```python
from build123d import *

# Parameters (mm, degrees)
SKETCH1_R           = 2.5
BOSS_EXTRUDE1_DEPTH = 15
CUT_EXTRUDE1_DEPTH  = 10


with BuildPart() as part:
    # Sketch1 → Boss-Extrude1 (new body, symmetric)
    with BuildSketch(Plane.XY):
        Circle(SKETCH1_R)
    extrude(amount=BOSS_EXTRUDE1_DEPTH, both=True)

    # Sketch2 → Cut-Extrude1 (cut)
    with BuildSketch(Plane(origin=(0, 0, -15), x_dir=(-1, 0, 0), z_dir=(0, 0, -1))):
        with BuildLine():
            Line((-0.5, -2.449489743), (-0.5, -1.949489743))
            Line((-0.5, -1.949489743), (0.5, -1.949489743))
            Line((0.5, -1.949489743), (0.5, -2.449489743))
            ThreePointArc((0.5, -2.449489743), (0, -2.5), (-0.5, -2.449489743))
        make_face()
    extrude(amount=-CUT_EXTRUDE1_DEPTH, mode=Mode.SUBTRACT)


solid = part.part
```
Input: part model. Units: mm. Frame: model coordinates. Coordinates: 2 decimals unless noted, no trailing zeros. Order: outer loops, then holes, each group sorted by start corner. A loop starts at its lowest first (then second) coordinate and runs counter-clockwise, first axis right, second up. Notation, with made-up numbers: (41.5, 12) - (84.5, 12) arc R27 ccw to (84.5, 32) - close; hole circle Ø4 at (79, 17.5). An arc over 180 degrees is marked (long way). Put each result on its own line as item: value.
1. Line query: line 1 along Z through (x, y) = (-0.2, -2.05); line 2 along X through (y, z) = (-2.1, -12); line 3 along Y through (x, z) = (0.1, 3). Output: solid intervals per line, ascending.
Report:
line 1: z = -5 to 15
line 2: x = -1.36 to -0.5, 0.5 to 1.36
line 3: y = -2.5 to 2.5
2. Contact query for flat-ended pins moving along their axis: pin 1 Ø0.6 at (x, y) = (0, -2.5) entering from -Z; pin 2 Ø0.8 at (x, z) = (0, -8) entering from -Y. Output: stop coordinate, or through.
Report:
pin 1: stops at z = -5
pin 2: stops at y = -1.95
3. Cut plane A-A on x = 0.2. Return the cut outline in (y, z), then the cut area to 3 significant figures.
Report:
outline: (-2.49, -5) - (-1.95, -5) - (-1.95, -15) - (2.49, -15) - (2.49, 15) - (-2.49, 15) - close
area: 144 mm2
4. Cut plane D-D on x = 1.4. Return the cut outline in (y, z).
Report:
outline: (-2.07, -15) - (2.07, -15) - (2.07, 15) - (-2.07, 15) - close
5. Draft query along X for faces 1 (the face through (-0.54, -2.44, 0.21)), 2 (the face through (0, -1.949, -10)), 3 (the face through (0, 0, -15)). Return one class per face: pulls with the +X half, pulls with the -X half, needs draft (parallel to the pull), parting line crosses it, or undercut.
Report:
face 1: parting line crosses it
face 2: undercut
face 3: needs draft
6. Cut plane C-C on y = -0.9. Return the cut outline in (x, z), then the cut area to 3 significant figures.
Report:
outline: (-2.33, -15) - (2.33, -15) - (2.33, 15) - (-2.33, 15) - close
area: 140 mm2
7. Cut plane B-B on z = 1.75. Return the cut outline in (x, y).
Report:
outline: circle Ø5 at (0, 0)
